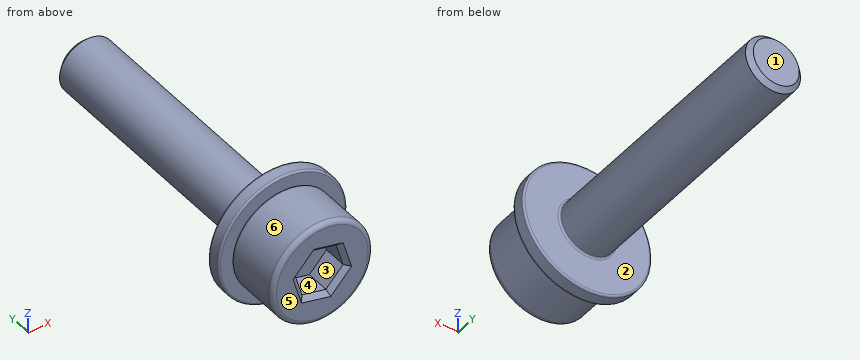
```python
from build123d import *

# Parameters (mm, degrees)
SKETCH1_R           = 2.75
BOSS_EXTRUDE1_DEPTH = 3
SKETCH2_R           = 1.5
BOSS_EXTRUDE2_DEPTH = 15
CUT_EXTRUDE1_DEPTH  = 1.5
CHAMFER1_SIZE       = 0.25
FILLET1_R           = 0.25
CHAMFER2_SIZE       = 0.25
FILLET2_R           = 0.1
SKETCH4_R           = 3.5
SKETCH4_R_2         = 1.5
BOSS_EXTRUDE3_DEPTH = 0.75
FILLET3_R           = 0.1


with BuildPart() as part:
    # Sketch1 → Boss-Extrude1 (new body)
    with BuildSketch(Plane(origin=(0, 0, 0), x_dir=(1, 0, 0), z_dir=(0, 1, 0))):
        with Locations(Location((0, 0, 0), (0, 0, 270))):
            Circle(SKETCH1_R)
    extrude(amount=BOSS_EXTRUDE1_DEPTH)

    # Sketch2 → Boss-Extrude2 (add)
    with BuildSketch(Plane(origin=(0, 3, 0), x_dir=(1, 0, 0), z_dir=(0, 1, 0))):
        with Locations(Location((0, 0, 0), (0, 0, 270))):
            Circle(SKETCH2_R)
    extrude(amount=BOSS_EXTRUDE2_DEPTH)

    # Sketch3 → Cut-Extrude1 (cut)
    with BuildSketch(Plane.XZ):
        Polygon((0.934168857, 0.974591477), (-0.376936549, 1.2963097), (-1.311105406, 0.321718223), (-0.934168857, -0.974591477), (0.376936549, -1.2963097), (1.311105406, -0.321718223), align=None)
    extrude(amount=-CUT_EXTRUDE1_DEPTH, mode=Mode.SUBTRACT)

    # Chamfer1
    chamfer1_edges = [part.edges().sort_by_distance(p)[0] for p in [
        (1.122637131, 0, 0.326436627),
        (0.278616154, 0, 1.135450588),
        (-0.844020977, 0, 0.809013962),
        (-1.122637131, 0, -0.326436627),
        (-0.278616154, 0, -1.135450588),
        (0.844020977, 0, -0.809013962),
    ]]
    chamfer(chamfer1_edges, length=CHAMFER1_SIZE)

    # Fillet1
    fillet1_edges = [part.edges().sort_by_distance(p)[0] for p in [
        (0, 0, -2.75),
    ]]
    fillet(fillet1_edges, radius=FILLET1_R)

    # Chamfer2
    chamfer2_edges = [part.edges().sort_by_distance(p)[0] for p in [
        (0, 18, -1.5),
    ]]
    chamfer(chamfer2_edges, length=CHAMFER2_SIZE)

    # Fillet2
    fillet2_edges = [part.edges().sort_by_distance(p)[0] for p in [
        (0, 3, -2.75),
    ]]
    fillet(fillet2_edges, radius=FILLET2_R)

    # Sketch4 → Boss-Extrude3 (add)
    with BuildSketch(Plane(origin=(0, 3, 0), x_dir=(1, 0, 0), z_dir=(0, 1, 0))):
        with Locations(Location((0, 0, 0), (0, 0, 270))):
            Circle(SKETCH4_R)
        with Locations(Location((0, 0, 0), (0, 0, 270))):
            Circle(SKETCH4_R_2, mode=Mode.SUBTRACT)
    extrude(amount=BOSS_EXTRUDE3_DEPTH)

    # Fillet3
    fillet3_edges = [part.edges().sort_by_distance(p)[0] for p in [
        (0, 3.75, -3.5),
        (0, 3, -3.5),
        (0, 3.75, -1.5),
    ]]
    fillet(fillet3_edges, radius=FILLET3_R)


solid = part.part
```
Could you check a few things on this model? Use its own coordinates, in mm. Face numbers are marked on the shaded views. A direction names the side the tool comes from. Round coordinates to 2 decimals unless told otherwise and drop trailing zeros. Loops run counter-clockwise (first coordinate to the right, second up) from the corner with the lowest first, then second, coordinate; pieces in that order, holes last. Notation, with made-up numbers: (44.25, -35) - (71.25, -35) arc R28 ccw to (71.25, -3) - close; hole circle Ø2 at (36, 11.5). An arc over 180 degrees is marked (long way). Answer in a Markdown table with one row per item. Add a question column.
(1) For the marked faces 1, 2 and 3, which set-ups out of +Z, -Z, +X, -X, +Y, -Y let a thin tool reach every point of the face, with its end or its side?
(2) If we mould it in two halves opening along Z, with no side actions, what happens to the marked faces 4, 5 and 6? For each: pulls with the +Z half, pulls with the -Z half, needs draft (parallel to the pull), parting line crosses it, or undercut.
(3) I need wall thicknesses on line 1 along Y through (x, z) = (1.25, -3); line 2 along Y through (x, z) = (-1.5, -0.75); line 3 along X through (y, z) = (9, 0). Which ranges of each line are inside material? Lowest first, please.
(4) If we section it at C-C (y = 5.5): Please give me the cut outline in (x, z).
(5) I'm going to push flat-ended pins straight in: pin 1 (1 mm diameter, centred on x = 0, z = 2.5, fed in from +Y); pin 2 (2 mm diameter, centred on y = 11.5, z = -1, fed in from +X); pin 3 (1 mm diameter, centred on y = 8.5, z = 1, fed in from +X). Where does each tip first touch, or does it pass through?
Model answer:
| question | item | result |
|---|---|---|
| 1 | face 1 | +Z, -Z, +X, -X, +Y |
| 1 | face 2 | +Y |
| 1 | face 3 | -Y |
| 2 | face 4 | undercut |
| 2 | face 5 | needs draft |
| 2 | face 6 | parting line crosses it |
| 3 | line 1 | y = 3 to 3.75 |
| 3 | line 2 | y = 0 to 3.75 |
| 3 | line 3 | x = -1.5 to 1.5 |
| 4 | outline | circle Ø3 at (0, 0) |
| 5 | pin 1 | stops at y = 3.75 |
| 5 | pin 2 | stops at x = 1.5 |
| 5 | pin 3 | stops at x = 1.41 |
